from build123d import *

# Parameters (mm, degrees)
SKETCH5_W               = 91.75
SKETCH5_H               = 67.75
SKETCH5_R               = 2.3876
SKETCH5_R_2             = 3.683
SKETCH5_R_3             = 1.5
SKETCH5_W_2             = 8.85
SKETCH5_H_2             = 31.2
SKETCH5_R_4             = 1.5875
BOSS_EXTRUDE1_DEPTH     = 6.35
F_8_32_TAPPED_HOLE1_D   = 3.4544
CUT_EXTRUDE2_START      = 3.175
SKETCH5_3_R             = 2.3876
SKETCH5_3_R_2           = 1.5875
CUT_EXTRUDE2_DEPTH      = 3.175
SKETCH8_W               = 25.4
SKETCH8_H               = 67.75
SKETCH8_R               = 1
BOSS_EXTRUDE2_DEPTH     = 6.35
F_1_4_20_TAPPED_HOLE2_D = 5.1054
CUT_EXTRUDE3_DEPTH      = 140.2958778
CUT_EXTRUDE3_DEPTH_BACK = 140.2958778
SKETCH11_R              = 2.032
CUT_EXTRUDE4_DEPTH      = 140.2958778
CUT_EXTRUDE4_DEPTH_BACK = 140.2958778
SKETCH12_W              = 0.25
SKETCH12_H              = 31.2
SKETCH12_H_2            = 31.222616973
FILLET2_R               = 1


with BuildPart() as part:
    # Sketch5 → Boss-Extrude1 (new body)
    # profile 1 of 6: a face of its own
    with BuildSketch(Plane.XY):
        with Locations((-48.669, 36.669)):
            Rectangle(SKETCH5_W, SKETCH5_H)
        with Locations((-7.874, 18.034)):
            Circle(SKETCH5_R, mode=Mode.SUBTRACT)
        with Locations((-7.874, 59.944)):
            Circle(SKETCH5_R, mode=Mode.SUBTRACT)
        with Locations((-18.034, 7.874)):
            Circle(SKETCH5_R, mode=Mode.SUBTRACT)
        with Locations((-59.944, 7.874)):
            Circle(SKETCH5_R, mode=Mode.SUBTRACT)
        with Locations((-19.9136, 19.9136)):
            Circle(SKETCH5_R_2, mode=Mode.SUBTRACT)
        with Locations((-52.794, 42.794)):
            Circle(SKETCH5_R_3, mode=Mode.SUBTRACT)
        with Locations((-78.119, 42.794)):
            Rectangle(SKETCH5_W_2, SKETCH5_H_2, mode=Mode.SUBTRACT)
        with Locations((-27.469, 42.794)):
            Rectangle(SKETCH5_W_2, SKETCH5_H_2, mode=Mode.SUBTRACT)
    # profile 2 of 6: a face of its own
    with BuildSketch(Plane.XY):
        with Locations((-7.874, 59.944)):
            Circle(SKETCH5_R)
        with Locations((-7.874, 59.944)):
            Circle(SKETCH5_R_4, mode=Mode.SUBTRACT)
    # profile 3 of 6: a face of its own
    with BuildSketch(Plane.XY):
        with Locations((-19.9136, 19.9136)):
            Circle(SKETCH5_R_2)
    # profile 4 of 6: a face of its own
    with BuildSketch(Plane.XY):
        with Locations((-7.874, 18.034)):
            Circle(SKETCH5_R)
        with Locations((-7.874, 18.034)):
            Circle(SKETCH5_R_4, mode=Mode.SUBTRACT)
    # profile 5 of 6: a face of its own
    with BuildSketch(Plane.XY):
        with Locations((-18.034, 7.874)):
            Circle(SKETCH5_R)
        with Locations((-18.034, 7.874)):
            Circle(SKETCH5_R_4, mode=Mode.SUBTRACT)
    # profile 6 of 6: a face of its own
    with BuildSketch(Plane.XY):
        with Locations((-59.944, 7.874)):
            Circle(SKETCH5_R)
        with Locations((-59.944, 7.874)):
            Circle(SKETCH5_R_4, mode=Mode.SUBTRACT)
    extrude(amount=BOSS_EXTRUDE1_DEPTH)

    # #8-32 Tapped Hole1 (through all)
    with Locations(Plane(origin=(-70.828, 42.794, 6.35), x_dir=(1, 0, 0), z_dir=(0, 0, 1))):
        with Locations((0, 0), (36.068, 0)):
            Hole(F_8_32_TAPPED_HOLE1_D / 2)

    # Sketch5<3> → Cut-Extrude2 (cut)
    # profile 1 of 4: a face of its own
    with BuildSketch(Plane.XY.offset(CUT_EXTRUDE2_START)):
        with Locations((-18.034, 7.874)):
            Circle(SKETCH5_3_R)
        with Locations((-18.034, 7.874)):
            Circle(SKETCH5_3_R_2, mode=Mode.SUBTRACT)
    # profile 2 of 4: a face of its own
    with BuildSketch(Plane.XY.offset(CUT_EXTRUDE2_START)):
        with Locations((-7.874, 18.034)):
            Circle(SKETCH5_3_R)
        with Locations((-7.874, 18.034)):
            Circle(SKETCH5_3_R_2, mode=Mode.SUBTRACT)
    # profile 3 of 4: a face of its own
    with BuildSketch(Plane.XY.offset(CUT_EXTRUDE2_START)):
        with Locations((-59.944, 7.874)):
            Circle(SKETCH5_3_R)
        with Locations((-59.944, 7.874)):
            Circle(SKETCH5_3_R_2, mode=Mode.SUBTRACT)
    # profile 4 of 4: a face of its own
    with BuildSketch(Plane.XY.offset(CUT_EXTRUDE2_START)):
        with Locations((-7.874, 59.944)):
            Circle(SKETCH5_3_R)
        with Locations((-7.874, 59.944)):
            Circle(SKETCH5_3_R_2, mode=Mode.SUBTRACT)
    extrude(amount=CUT_EXTRUDE2_DEPTH, mode=Mode.SUBTRACT)

    # Sketch8 → Boss-Extrude2 (add)
    with BuildSketch(Plane.XY):
        with Locations((-107.244, 36.669)):
            Rectangle(SKETCH8_W, SKETCH8_H)
        with Locations((-112.944, 7.794)):
            Circle(SKETCH8_R, mode=Mode.SUBTRACT)
    extrude(amount=BOSS_EXTRUDE2_DEPTH)

    # 1/4-20 Tapped Hole2 (through all)
    with Locations(Plane(origin=(-112.944, 7.794, 6.35), x_dir=(1, 0, 0), z_dir=(0, 0, 1))):
        with Locations((0, 0)):
            Hole(F_1_4_20_TAPPED_HOLE2_D / 2)

    # Sketch11 → Cut-Extrude3 (cut, two sides: drawn at the far end of the back side and taken through both)
    with BuildSketch(Plane.XY.offset(6.35).offset(-CUT_EXTRUDE3_DEPTH_BACK)):
        with Locations((-69.544, 61.044)):
            Circle(SKETCH11_R)
        with Locations((-36.044, 61.044)):
            Circle(SKETCH11_R)
        with Locations((-36.044, 24.544)):
            Circle(SKETCH11_R)
        with Locations((-69.544, 24.544)):
            Circle(SKETCH11_R)
    extrude(amount=CUT_EXTRUDE3_DEPTH + CUT_EXTRUDE3_DEPTH_BACK, mode=Mode.SUBTRACT)

    # Sketch12 → Cut-Extrude4 (cut, two sides: drawn at the far end of the back side and taken through both)
    with BuildSketch(Plane.XY.offset(6.35).offset(-CUT_EXTRUDE4_DEPTH_BACK)):
        with Locations((-32.019, 42.794)):
            Rectangle(SKETCH12_W, SKETCH12_H)
        with Locations((-73.569, 42.782691514)):
            Rectangle(SKETCH12_W, SKETCH12_H_2)
    extrude(amount=CUT_EXTRUDE4_DEPTH + CUT_EXTRUDE4_DEPTH_BACK, mode=Mode.SUBTRACT)

    # Fillet2
    fillet2_edges = [part.edges().sort_by_distance(p)[0] for p in [
        (-119.944, 70.544, 3.175),
        (-2.794, 2.794, 3.175),
        (-2.794, 70.544, 3.175),
        (-119.944, 2.794, 3.175),
    ]]
    fillet(fillet2_edges, radius=FILLET2_R)


solid = part.part
Verification items for the finished model (mm, model axes). A direction names the side the tool comes from. Round coordinates to 2 decimals unless told otherwise and drop trailing zeros. Order: outer loops, then holes, each group sorted by start corner. A loop starts at its lowest first (then second) coordinate and runs counter-clockwise, first axis right, second up.
1. Access from +Z, -Z, +X, -X, +Y, -Y to the whole of each face (thin tool, end or side, straight path). Record for faces 4 (the cylindrical face through (-57.74, 6.96, 4.74)), 5 (the flat face through (-78, 27.194, 3)), 6 (the flat face through (-62, 2.794, 3)).
Final values:
face 4: +Z
face 5: +Z, -Z
face 6: +Z, -Z, +X, -X, -Y
2. Release check for a two-part mould opening along X. For faces 1 (the flat face through (-62, 37, 0)), 2 (the cylindrical face through (-38.074, 24.633, 3.131)), 3 (the cylindrical face through (-110.394, 7.906, 3.131)) record: +X half, -X half, draft (parallel to the pull), parting line (faces both ways), or undercut.
Final values:
face 1: draft
face 2: undercut
face 3: undercut
3. Section check A-A on y = 37.5. Record the cut outline in (x, z).
Final values:
outline: (-119.94, 0) - (-82.54, 0) - (-82.54, 6.35) - (-119.94, 6.35) - close; (-73.44, 0) - (-32.14, 0) - (-32.14, 6.35) - (-73.44, 6.35) - close; (-23.04, 0) - (-2.79, 0) - (-2.79, 6.35) - (-23.04, 6.35) - close
4. Thickness scan on L1, parallel to X at y = 29.5, z = 2.25; L2, parallel to X at y = 44, z = 3.5; L3, parallel to X at y = 60.5, z = 0.75. Record the ranges inside material, lowest first.
Final values:
L1: x = -119.94 to -82.54, -73.44 to -32.14, -23.04 to -2.79
L2: x = -119.94 to -82.54, -73.44 to -72.06, -69.59 to -53.69, -51.9 to -36, -33.52 to -32.14, -23.04 to -2.79
L3: x = -119.94 to -71.5, -67.59 to -38, -34.09 to -9.36, -6.39 to -2.79
5. Go/stop test with flat-tipped pins: P1, Ø2.5, axis at x = -52.794, y = 42.794, coming from the +Z side; P2, Ø2.5, axis at x = -8.5, y = 18, coming from the +Z side (3 decimals). Record where each tip stops, or that it passes through.
Final values:
P1: passes through
P2: stops at z = 3.175
6. Section check B-B on z = 2. State how many separate pieces and enclosed holes the cut face has, then the cut area to 3 significant figures.
Final values:
separate pieces: 1
enclosed holes: 14
area: 7,240 mm2
